Autodesk Fusion 360 part; units mm, degrees
sketch "Sketch1" plane through (0, 0, 0) normal (0, 1, 0) x (1, 0, 0)
  circle A0 centre (0, 0) radius 20
  circle A1 centre (-55, 0) radius 16 construction
  circle A2 centre (-55, 0) radius 11
  line L0 (0, 0) -> (-55, 0) construction
  line L1 (-85, 30) -> (90, 30)
  line L2 (90, 30) -> (90, -30)
  line L3 (90, -30) -> (-85, -30)
  line L4 (-85, -30) -> (-85, 30)
  line L5 (-40, 30) -> (-40, -30)
  line L6 (-66.3137, -11.3137) -> (-43.6863, 11.3137) construction
  line L7 (-66.3137, 11.3137) -> (-43.6863, -11.3137) construction
  line L8 (-55, 16) -> (-55, -16) construction
  line L9 (38.43, -23.57) -> (85.57, -23.57) construction
  line L10 (85.57, -23.57) -> (85.57, 23.57) construction
  line L11 (85.57, 23.57) -> (38.43, 23.57) construction
  line L12 (38.43, 23.57) -> (38.43, -23.57) construction
  line L13 (38.43, 23.57) -> (85.57, -23.57) construction
  circle A3 centre (62, 0) radius 19.5
  point P0 (-66.3137, 11.3137)
  point P1 (-55, 16)
  point P2 (-43.6863, 11.3137)
  point P3 (-43.6863, -11.3137)
  point P4 (-55, -16)
  point P5 (-66.3137, -11.3137)
  dimension "d1" = 32
  dimension "d2" = 22
  dimension "d3" = 55
  dimension "d4" = 40
  dimension "d5" = 60
  dimension "d6" = 30
  dimension "d7" = 90
  dimension "d8" = 15
  dimension "d9" = 45
  dimension "d20" = 47.14
  dimension "d22" = 39
  dimension "d27" = 62
extrude "Extrude1" add sketch "Sketch1" along normal blind 25
extrude "Extrude3" cut sketch "Sketch1" along normal blind 15 contours L1 L2 L3 L5 | A3
hole "Hole1" at (-66.3137, 0, 11.3137) at (-55, 0, 16) at (-66.3137, 0, -11.3137) at (-55, 0, -16) at (-43.6863, 0, -11.3137) at (-43.6863, 0, 11.3137) direction (0, 1, 0) diameter 3.332 depth 15 tip angle 118
hole "Hole2" at (38.43, 0, 23.57) at (38.43, 0, -23.57) at (85.57, 0, 23.57) at (85.57, 0, -23.57) direction (0, -1, 0) diameter 4.234 depth 60 tip angle 118
chamfer "Chamfer1" distance 5 angle 45 4 edges at (-85, 12.5, -30) (-85, 12.5, 30) (90, 20, -30) (90, 20, 30)
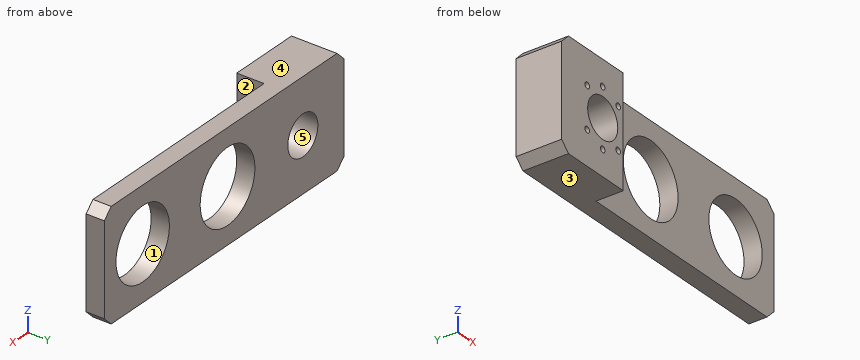
Source: CAD feature listing. Evaluate the final solid. Frame: model axes, mm. Face numbers are marked on the shaded views. A direction names the side the tool comes from. Round coordinates to 2 decimals unless told otherwise and drop trailing zeros. Loops run counter-clockwise (first coordinate to the right, second up) from the corner with the lowest first, then second, coordinate; pieces in that order, holes last. Notation, with made-up numbers: M 71.5,87.5 L 126.5,87.5 A23 cw 126.5,119.5 Z; hole C 66,-19.5 d10. An arc over 180 degrees is marked long. Use a Markdown table: item, result. Add a question column.
1. Line query: line 1 (X direction, y = 12.25, z = 11.5); line 2 (X direction, y = 17.75, z = 0); line 3 (X direction, y = 19.75, z = 9). Output: solid intervals per line, ascending.
2. Reachability of the marked faces 1 and 2 from +Z, -Z, +X, -X, +Y, -Y: full face, straight path, thin tool, end or side. Return the list, or none.
3. Section query D-D on x = 0. Return the cut outline in (y, z).
4. Mould query, pull axis Z, two halves, no side actions, for the marked faces 3, 4 and 5. Classes: pulls with the +Z half, pulls with the -Z half, needs draft (parallel to the pull), parting line crosses it, or undercut.
5. Section query A-A on x = 62. Return the cut outline in (y, z), then the cut area to 3 significant figures.
6. Contact query for flat-ended pins moving along their axis: P1, Ø10, axis at x = -15.5, y = 7.5, coming from the -Z side; P2, Ø1, axis at y = 6, z = -5, coming from the +X side; P3, Ø2, axis at x = -43.69, z = -11.31, coming from the -Y side; P4, Ø2.5, axis at x = -66.31, z = -11.31, coming from the -Y side. Output: stop coordinate, or through.
7. Section query B-B on y = 21. Return the cut outline in (x, z).
8. Section query C-C on z = 2. Return the cut outline in (x, y), then the cut area to 3 significant figures.
Reported:
| question | item | result |
|---|---|---|
| 1 | line 1 | x = -85 to -67.97, -64.66 to -45.34, -42.03 to -40 |
| 1 | line 2 | x = -85 to -66, -44 to -20, 20 to 42.5, 81.5 to 90 |
| 1 | line 3 | x = -85 to -61.32, -48.68 to -17.86, 17.86 to 44.7, 79.3 to 90 |
| 2 | face 1 | +Y, -Y |
| 2 | face 2 | +Z, -Z, +X, -Y |
| 3 | outline | M 15,-30 L 25,-30 L 25,-20 L 15,-20 Z; M 15,20 L 25,20 L 25,30 L 15,30 Z |
| 4 | face 3 | pulls with the -Z half |
| 4 | face 4 | pulls with the +Z half |
| 4 | face 5 | undercut |
| 5 | outline | M 15,-30 L 25,-30 L 25,-19.5 L 15,-19.5 Z; M 15,19.5 L 25,19.5 L 25,30 L 15,30 Z |
| 5 | area | 210 mm² |
| 6 | P1 | passes through |
| 6 | P2 | stops at x = -40 |
| 6 | P3 | stops at y = 15.4 |
| 6 | P4 | stops at y = 15.25 |
| 7 | outline | M -85,-25 L -80,-30 L 85,-30 L 90,-25 L 90,25 L 85,30 L -80,30 L -85,25 Z; hole C -55,0 d22; hole C 0,0 d40; hole C 62,0 d39 |
| 8 | outline | M -85,0 L -65.82,0 L -65.82,25 L -85,25 Z; M -44.18,0 L -40,0 L -40,15 L -19.9,15 L -19.9,25 L -44.18,25 Z; M 19.9,15 L 42.6,15 L 42.6,25 L 19.9,25 Z; M 81.4,15 L 90,15 L 90,25 L 81.4,25 Z |
| 8 | area | 1,100 mm² |
